```python
from build123d import *

# Parameters (mm, degrees)
BOSS_EXTRUDE1_DEPTH = 30
SKETCH2_W           = 20
SKETCH2_H           = 200
CUT_EXTRUDE1_DEPTH  = 260
SKETCH3_R           = 2.25
CUT_EXTRUDE2_DEPTH  = 71
SKETCH5_R           = 2.25
CUT_EXTRUDE3_DEPTH  = 71


with BuildPart() as part:
    # Sketch1 → Boss-Extrude1 (new body)
    with BuildSketch(Plane(origin=(0, 0, 0), x_dir=(0, 0, -1), z_dir=(1, 0, 0))):
        with BuildLine():
            Line((20, 0), (-20, 0))
            Line((-20, 0), (-20, 40))
            ThreePointArc((-20, 40), (0, 60), (20, 40))
            Line((20, 40), (20, 0))
        make_face()
    extrude(amount=BOSS_EXTRUDE1_DEPTH)

    # Sketch2 → Cut-Extrude1 (cut)
    with BuildSketch(Plane(origin=(0, 267.144833217, 0), x_dir=(1, 0, 0), z_dir=(0, 1, 0))):
        with Locations((15, 0)):
            Rectangle(SKETCH2_W, SKETCH2_H)
    extrude(amount=-CUT_EXTRUDE1_DEPTH, mode=Mode.SUBTRACT)

    # Sketch3 → Cut-Extrude2 (cut, through all)
    with BuildSketch(Plane.XZ):
        with Locations(Location((15, 0, 0), (0, 0, 270))):
            Circle(SKETCH3_R)
    extrude(amount=-CUT_EXTRUDE2_DEPTH, mode=Mode.SUBTRACT)

    # Sketch5 → Cut-Extrude3 (cut, through all)
    with BuildSketch(Plane(origin=(30, 0, 0), x_dir=(0, 0, -1), z_dir=(1, 0, 0))):
        with Locations((0, 40)):
            Circle(SKETCH5_R)
    extrude(amount=-CUT_EXTRUDE3_DEPTH, mode=Mode.SUBTRACT)


solid = part.part
```
Geometry check sheet. Reference: the model listing, model coordinates, mm. A direction names the side the tool comes from. Coordinates: 2 decimals unless noted, no trailing zeros. Order: outer loops, then holes, each group sorted by start corner. A loop starts at its lowest first (then second) coordinate and runs counter-clockwise, first axis right, second up.
Item 1: Section check C-C (x = 15.75). Enter the section's corners in (y, z), plus the area to 3 significant figures.
Item 2: Mould release check, pull along Z, two halves, no side actions. Record for faces 3 (the flat face through (4.8, 15.3, 20)), 4 (the flat face through (30, 30, 0)), 5 (the cylindrical face through (27.54, 42.23, 0.29)): released by +Z, released by -Z, zero draft, split by the parting line, or undercut.
Item 3: Section check B-B (z = 0). Enter the section's corners in (x, y), plus the area to 3 significant figures.
Item 4: Depth check by flat-ended pin: pin 1 (5 mm diameter, centred on x = 23, y = 42, fed in from +Z); pin 2 (12 mm diameter, centred on x = 26.5, z = 7, fed in from +Y) (3 decimals); pin 3 (10 mm diameter, centred on x = 15.5, z = -2, fed in from +Y). Enter the tip coordinate at first touch or a pass-through.
Item 5: Section check D-D (z = 16). Enter the section's corners in (x, y), plus the area to 3 significant figures.
Item 6: Section check A-A (y = 52). Enter the section's corners in (x, z).
Item 7: Scan lines: line 1 along X through (y, z) = (5, 0); line 2 along X through (y, z) = (15, -5); line 3 along Y through (x, z) = (28.95, 0). Record each from-to range of solid material in increasing order.
Item 8: Tool access check on faces 1 (the cylindrical face through (12.804, 3.522, 0.488)), 2 (the flat face through (12.6, 7.145, -0.3)). Record the directions out of +Z, -Z, +X, -X, +Y, -Y that give a thin tool (end or side, any length) a straight path to the whole face; none if there is none.
Check sheet entries:
1. outline: (0, -20) - (7.14, -20) - (7.14, -2.12) - (0, -2.12) - close; (0, 2.12) - (7.14, 2.12) - (7.14, 20) - (0, 20) - close
1. area: 255 mm2
2. face 3: released by +Z
2. face 4: zero draft
2. face 5: undercut
3. outline: (0, 0) - (12.75, 0) - (12.75, 7.14) - (5, 7.14) - (5, 37.75) - (0, 37.75) - close; (0, 42.25) - (5, 42.25) - (5, 60) - (0, 60) - close; (17.25, 0) - (30, 0) - (30, 37.75) - (25, 37.75) - (25, 7.14) - (17.25, 7.14) - close; (25, 42.25) - (30, 42.25) - (30, 60) - (25, 60) - close
3. area: 666 mm2
4. pin 1: stops at z = 19.99
4. pin 2: stops at y = 59.975
4. pin 3: stops at y = 7.14
5. outline: (0, 0) - (30, 0) - (30, 52) - (25, 52) - (25, 7.14) - (5, 7.14) - (5, 52) - (0, 52) - close
5. area: 663 mm2
6. outline: (0, -16) - (5, -16) - (5, 16) - (0, 16) - close; (25, -16) - (30, -16) - (30, 16) - (25, 16) - close
7. line 1: x = 0 to 12.75, 17.25 to 30
7. line 2: x = 0 to 5, 25 to 30
7. line 3: y = 0 to 37.75, 42.25 to 60
8. face 1: +Y, -Y
8. face 2: +Z, -Z, +Y
